from build123d import *

# Parameters (mm, degrees)
SKETCH1_W                       = 20
SKETCH1_H                       = 10
BOSS_EXTRUDE1_DEPTH             = 10
CUT_EXTRUDE1_DEPTH              = 10
SKETCH3_W                       = 20
SKETCH3_H                       = 4
BOSS_EXTRUDE2_DEPTH             = 15
TAP_DRILL_FOR_M3X0_5_TAP6_D     = 3.35
TAP_DRILL_FOR_M3X0_5_TAP6_DEPTH = 4


with BuildPart() as part:
    # Sketch1 → Boss-Extrude1 (new body)
    with BuildSketch(Plane.XY):
        Rectangle(SKETCH1_W, SKETCH1_H)
    extrude(amount=BOSS_EXTRUDE1_DEPTH)

    # Sketch2 → Cut-Extrude1 (cut)
    with BuildSketch(Plane(origin=(0, 5, 0), x_dir=(1, 0, 0), z_dir=(0, 1, 0))):
        with BuildLine():
            Line((-10, -10), (10, -10))
            ThreePointArc((10, -10), (0, -7.320508076), (-10, -10))
        make_face()
    extrude(amount=-CUT_EXTRUDE1_DEPTH, mode=Mode.SUBTRACT)

    # Sketch3 → Boss-Extrude2 (add)
    with BuildSketch(Plane(origin=(0, 0, 0), x_dir=(-1, 0, 0), z_dir=(0, 0, -1))):
        Rectangle(SKETCH3_W, SKETCH3_H)
    extrude(amount=BOSS_EXTRUDE2_DEPTH)

    # Tap Drill for M3x0.5 Tap6
    with Locations(Plane(origin=(0, 2, 0), x_dir=(1, 0, 0), z_dir=(0, 1, 0))):
        with Locations((0, 11)):
            Hole(TAP_DRILL_FOR_M3X0_5_TAP6_D / 2, depth=TAP_DRILL_FOR_M3X0_5_TAP6_DEPTH)


solid = part.part
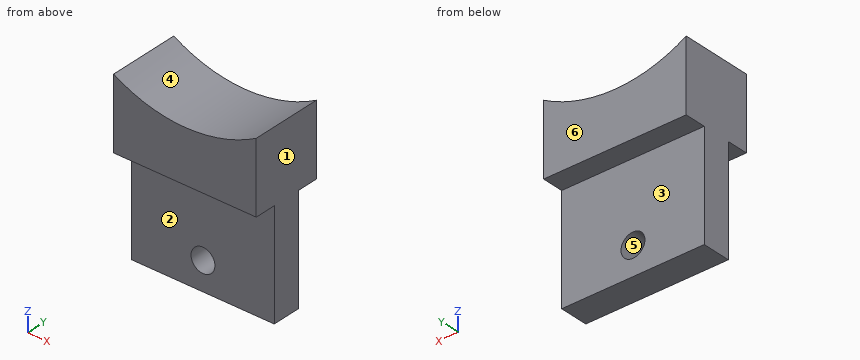
CAD build for the part. Positions are in the model's coordinates, mm. Face numbers are marked on the shaded views. A direction names the side the tool comes from. Give positions to 0.01 mm unless a question says otherwise; leave off trailing zeros. Loops run counter-clockwise (first coordinate to the right, second up) from the corner with the lowest first, then second, coordinate; pieces in that order, holes last. Notation, with made-up numbers: M 75.5,20.5 L 122.5,20.5 A17 cw 122.5,45.5 Z; hole C 86,-24 d3. An arc over 180 degrees is marked long. Write each question's results on one line, items separated by ' | '.
Q1. Mould opens along Z. For the marked faces 4, 5 and 6 say: pulls with the +Z half, pulls with the -Z half, needs draft (parallel to the pull), parting line crosses it, or undercut.
Geometry check:
face 4: pulls with the +Z half | face 5: undercut | face 6: needs draft
Q2. Band-saw the part on A-A on x = 0. Write the cut outline in (y, z) (1 decimal), and give its area (3 significant figures).
Geometry check:
outline: M -5,0 L -2,0 L -2,-9.3 L 2,-9.3 L 2,0 L 5,0 L 5,7.3 L -5,7.3 Z; M -2,-15 L 2,-15 L 2,-12.7 L -2,-12.7 Z | area: 120 mm²
Q3. Band-saw the part on D-D on x = -3.25. Write the cut outline in (y, z), and give its area (3 significant figures).
Geometry check:
outline: M -5,0 L -2,0 L -2,-15 L 2,-15 L 2,0 L 5,0 L 5,7.59 L -5,7.59 Z | area: 136 mm²
Q4. Probe probe 1 along Z at (x, y) = (0, -0.55) (1 decimal); probe 2 along X at (y, z) = (0.35, -11) (3 decimals); probe 3 along Y at (x, z) = (5.25, -4.75). List the from-to ranges inside material, lowest first.
Geometry check:
probe 1: z = -15 to -12.7, -9.3 to 7.3 | probe 2: x = -10 to -1.675, 1.675 to 10 | probe 3: y = -2 to 2
Q5. Flat gauge pins, fed straight in: P1, Ø0.9, axis at x = 2.5, y = 3, coming from the -Z side; P2, Ø1.5, axis at x = 1, z = -8, coming from the +Y side; P3, Ø3, axis at x = -8, y = -2.5, coming from the +Z side. Where does each tip first touch, or does it go through?
Geometry check:
P1: stops at z = 0 | P2: stops at y = 2 | P3: stops at z = 9.72
Q6. Band-saw the part on B-B on z = -11. Write the cut outline in (x, y) (3 decimals), and give its area (3 significant figures).
Geometry check:
outline: M -10,-2 L -1.675,-2 L -1.675,2 L -10,2 Z; M 1.675,-2 L 10,-2 L 10,2 L 1.675,2 Z | area: 66.6 mm²
Q7. Which spindle directions (+Z, -Z, +X, -X, +Y, -Y) get a long thin tool onto all of the face, cutting with end or side? Do the marked faces 1, 2 and 3. Say none if no direction does.
Geometry check:
face 1: +Z, -Z, +X, +Y, -Y | face 2: -Z, +X, -X, -Y | face 3: -Z, +X, -X, +Y
